The listing builds one solid part. Answer for the finished solid, in the listing's coordinates (mm). A direction names the side the tool comes from. Coordinates: 2 decimals unless noted, no trailing zeros. Write each loop counter-clockwise with the first axis right and the second up, starting at its lowest first coordinate (ties: lowest second). Pieces come first, ordered by that corner, then holes.
(1) Straight lines are drawn through the part: line 1 (Z direction, x = -1, y = -48); line 2 (Y direction, x = 16, z = -63); line 3 (X direction, y = -5.5, z = -74). For each, find the intervals that lie inside material, in ascending order.
(2) Given P1, Ø3, axis at y = -59.5, z = 24, coming from the +X side; P2, Ø12, axis at x = 0.5, z = 19.5, coming from the +Y side; P3, Ø6, axis at x = 12, y = -38, coming from the +Z side, each flat-ended and moving along its own axis, determine where each tip first touches the part or whether it passes through.
(3) Which of the six approach directions +Z, -Z, +X, -X, +Y, -Y give full straight-line access (tool end or side, diameter ignored) to faces 1 (the cylindrical face through (28.57, -15.34, -0.63)), 2 (the cylindrical face through (-5.506, -65.315, -24.796)), 3 (the flat face through (0, -107.95, 0)), 4 (the cylindrical face through (-28.57, -15.34, 0.63))?
(4) The part is cut by section A-A on y = -10. Determine the outline of the cut face in (x, z) (3 decimals), plus the area to 3 significant figures.
(5) The part is cut by section B-B on z = -44.5. Determine the outline of the cut face in (x, y).
from build123d import *

# Parameters (mm, degrees)
F0_R     = 28.575
F1_DEPTH = 25.4
F2_R     = 25.4
F3_DEPTH = 82.55
F4_R     = 25.4
F5_DEPTH = 107.95
F6_R     = 25.4
F7_DEPTH = 120.65
F8_R     = 1.5875


with BuildPart() as f1:
    # F0 (on Front) → F1 (new body)
    with BuildSketch(Plane.XZ):
        Circle(F0_R)
    extrude(amount=F1_DEPTH)

    # F2 (on face) → F3 (join)
    with BuildSketch(Plane.XZ.offset(25.4)):
        Circle(F2_R)
    extrude(amount=F3_DEPTH)

    # F4 (on Top) → F5 (join)
    with BuildSketch(Plane.XY):
        Circle(F4_R)
    extrude(amount=-F5_DEPTH)

    # F6 (on Top) → F7 (join)
    with BuildSketch(Plane.XY):
        Circle(F6_R)
    extrude(amount=F7_DEPTH)

    # F8
    f8_edges = [f1.edges().sort_by_distance(p)[0] for p in [
        (-25.4, -107.95, 0),
    ]]
    fillet(f8_edges, radius=F8_R)


solid = f1.part
Model answer:
1. line 1: z = -25.38 to 25.38
1. line 2: y = -19.73 to 19.73
1. line 3: x = -24.8 to 24.8
2. P1: stops at x = 11.79
2. P2: stops at y = 25.4
2. P3: stops at z = 23.75
3. face 1: +X, -Y
3. face 2: -Y
3. face 3: +Z, -Z, +X, -X, -Y
3. face 4: -X, -Y
4. outline: (-23.349, -107.95) - (23.349, -107.95) - (23.349, -16.473) arc R28.575 ccw to (23.349, 16.473) - (23.349, 120.65) - (-23.349, 120.65) - (-23.349, 16.473) arc R28.575 ccw to (-23.349, -16.473) - close
4. area: 10,900 mm2
5. outline: circle Ø50.8 at (0, 0)
